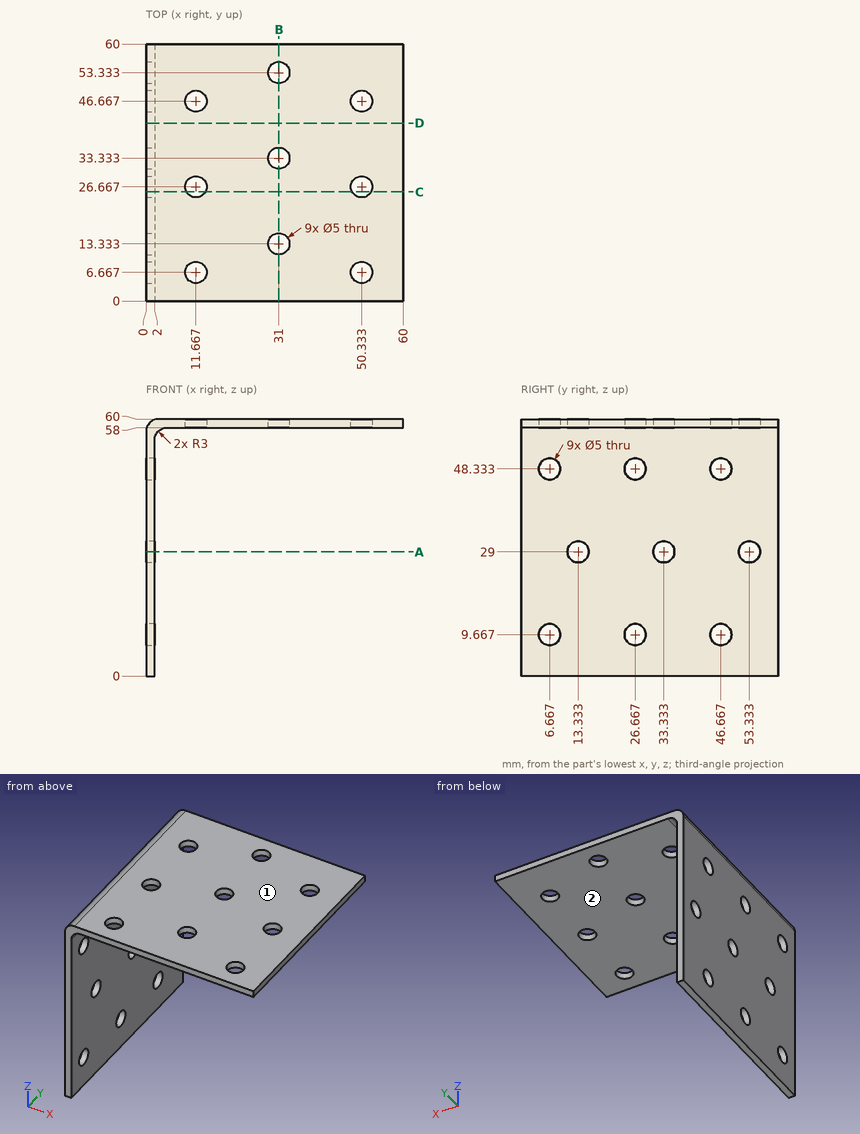
Study the drawing (mm; zero at the part's minimum x, y, z) and answer. A direction names the side the tool comes from. Coordinates: 2 decimals unless noted, no trailing zeros. Write each loop counter-clockwise with the first axis right and the second up, starting at its lowest first coordinate (ties: lowest second). Pieces come first, ordered by that corner, then holes. Notation, with made-up numbers: (19, -30.75) - (63, -30.75) arc R25 ccw to (63, 7.25) - close; hole circle Ø10 at (38.5, 7). An arc over 180 degrees is marked (long way). Answer as a JSON object with one key per item and string values. Group by question number.
1. A cutting plane is placed at A-A (z = 29). Determine the outline of the cut face in (x, y).
2. Consider L1, parallel to Y at x = 1.5, z = 29; L2, parallel to Z at x = 57, y = 3.5; L3, parallel to X at y = 37.5, z = 11. Determine where each line is inside the solid, lowest interval first. Write a range as [from, to].
3. A cutting plane is placed at C-C (y = 25.5). Determine the outline of the cut face in (x, z) (1 decimal).
4. Which of the six approach directions +Z, -Z, +X, -X, +Y, -Y give full straight-line access (tool end or side, diameter ignored) to the marked faces 1 and 2?
5. A cutting plane is placed at D-D (y = 41.5). Determine the outline of the cut face in (x, z), plus the area to 3 significant figures.
6. A cutting plane is placed at B-B (x = 31). Determine the outline of the cut face in (y, z).
7. Each of these flat-tipped pins is pushed along its axis until it touches: P1, Ø6.5, axis at y = 53.33, z = 29, coming from the +X side; P2, Ø8, axis at x = 11.67, y = 26.67, coming from the -Z side; P3, Ø4, axis at x = 31, y = 53.33, coming from the +Z side. Where does it stop, or does it pass through?
Worked out:
{
 "1": {"outline": "(0, 0) - (2, 0) - (2, 10.83) - (0, 10.83) - close; (0, 15.83) - (2, 15.83) - (2, 30.83) - (0, 30.83) - close; (0, 35.83) - (2, 35.83) - (2, 50.83) - (0, 50.83) - close; (0, 55.83) - (2, 55.83) - (2, 60) - (0, 60) - close"},
 "2": {"L1": "y = [0, 10.83], [15.83, 30.83], [35.83, 50.83], [55.83, 60]", "L2": "z = [58, 60]", "L3": "x = [0, 2]"},
 "3": {"outline": "(0, 0) - (2, 0) - (2, 7.5) - (0, 7.5) - close; (0, 11.9) - (2, 11.9) - (2, 46.1) - (0, 46.1) - close; (0, 50.5) - (2, 50.5) - (2, 55) arc R3 cw to (5, 58) - (9.5, 58) - (9.5, 60) - (3, 60) arc R3 ccw to (0, 57) - close; (13.9, 58) - (48.1, 58) - (48.1, 60) - (13.9, 60) - close; (52.5, 58) - (60, 58) - (60, 60) - (52.5, 60) - close"},
 "4": {"face 1": "+Z, +X, -X, +Y, -Y", "face 2": "-Z, +X, +Y, -Y"},
 "5": {"outline": "(0, 0) - (2, 0) - (2, 55) arc R3 cw to (5, 58) - (60, 58) - (60, 60) - (3, 60) arc R3 ccw to (0, 57) - close", "area": "236 mm²"},
 "6": {"outline": "(0, 58) - (10.83, 58) - (10.83, 60) - (0, 60) - close; (15.83, 58) - (30.83, 58) - (30.83, 60) - (15.83, 60) - close; (35.83, 58) - (50.83, 58) - (50.83, 60) - (35.83, 60) - close; (55.83, 58) - (60, 58) - (60, 60) - (55.83, 60) - close"},
 "7": {"P1": "stops at x = 2", "P2": "stops at z = 58", "P3": "passes through"}
}
